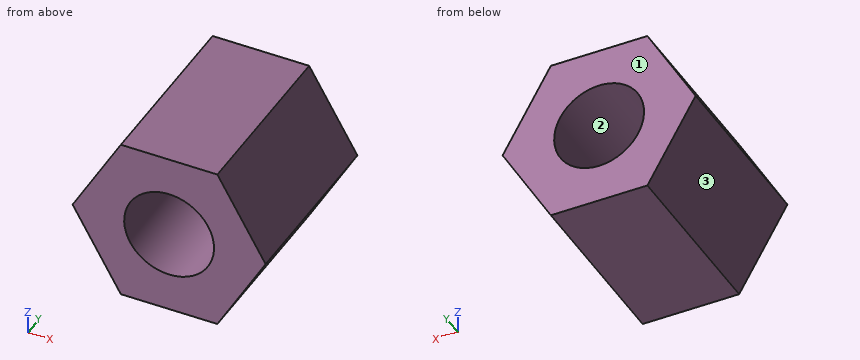
from build123d import *

# Parameters (mm, degrees)
EXTRUDE_1_DEPTH = 2.5


with BuildPart() as part:
    # 草图1 → 凸台-拉伸1 (new body, symmetric)
    with BuildSketch(Plane(origin=(0, 0, 0), x_dir=(1, 0, 0), z_dir=(0, 1, 0))):
        Polygon((2.684678752, 0), (1.342339376, 2.325), (-1.342339376, 2.325), (-2.684678752, 0), (-1.342339376, -2.325), (1.342339376, -2.325), align=None)
    extrude(amount=EXTRUDE_1_DEPTH, both=True)

    # 草图2 → M3 螺纹孔1 (revolve, cut)
    with BuildSketch(Plane(origin=(0, -2.5, 0), x_dir=(0, 0, -1), z_dir=(1, 0, 0))):
        Polygon((0, 0), (0, 8.251075774), (1.25, 7.5), (1.25, 0), align=None)
    hole_wizard_m3_1 = revolve(axis=Axis((0, -8.85, 0), (0, 1, 0)), mode=Mode.SUBTRACT)

    # 镜向1: M3 螺纹孔1 across plane
    add(hole_wizard_m3_1.mirror(Plane.ZX), mode=Mode.SUBTRACT)


solid = part.part
Design review of the part built by this model. Coordinates are the model's own, in mm. Face numbers are marked on the shaded views. Give positions to 0.01 mm unless a question says otherwise; leave off trailing zeros. Loops run counter-clockwise (first coordinate to the right, second up) from the corner with the lowest first, then second, coordinate; pieces in that order, holes last. Notation, with made-up numbers: (51.5, -32.5) - (91.5, -32.5) arc R14 cw to (91.5, -22.5) - close; hole circle Ø9 at (-34, 32). An arc over 180 degrees is marked (long way). Use CSV: the item, a comma, the result in double quotes. Start each with the question number.
1. Draft analysis for pull direction Z (two halves, no side actions). For the marked faces 1, 2 and 3, state which applies: released by +Z, released by -Z, zero draft, split by the parting line, or undercut.
2. Add section A-A (x = 0). State the section outline as (y, z) points (3 decimals), plus the area to 4 significant figures.
3. Wall thickness on L1, parallel to Z at x = 0, y = 0.75 (3 decimals); L2, parallel to X at y = -1.8, z = -0.75; L3, parallel to Z at x = -1, y = 1.65 (3 decimals): over which ranges is each line inside the solid? List them lowest first.
4. Add section B-B (y = 1.15). State the section outline as (x, z) points (3 decimals).
5. Add section C-C (z = -0.4). State the section outline as (x, y) points, plus the area to 3 significant figures.
6. Add section D-D (z = 1.7). State the section outline as (x, y) points, plus the area to 3 significant figures.
Results found:
1,face 1,"zero draft"
1,face 2,"undercut"
1,face 3,"released by -Z"
2,outline,"(-2.5, -2.325) - (2.5, -2.325) - (2.5, -1.25) - (-2.5, -1.25) - close; (-2.5, 1.25) - (2.5, 1.25) - (2.5, 2.325) - (-2.5, 2.325) - close"
2,area,"10.75 mm²"
3,L1,"z = -2.325 to -1.25, 1.25 to 2.325"
3,L2,"x = -2.25 to -1, 1 to 2.25"
3,L3,"z = -2.325 to -0.75, 0.75 to 2.325"
4,outline,"(-2.685, 0) - (-1.342, -2.325) - (1.342, -2.325) - (2.685, 0) - (1.342, 2.325) - (-1.342, 2.325) - close; hole circle Ø2.5 at (0, 0)"
5,outline,"(-2.45, -2.5) - (-1.18, -2.5) - (-1.18, 2.5) - (-2.45, 2.5) - close; (1.18, -2.5) - (2.45, -2.5) - (2.45, 2.5) - (1.18, 2.5) - close"
5,area,"12.7 mm²"
6,outline,"(-1.7, -2.5) - (1.7, -2.5) - (1.7, 2.5) - (-1.7, 2.5) - close"
6,area,"17.0 mm²"
